Source: CAD feature listing. Evaluate the final solid. Frame: model axes, mm. A direction names the side the tool comes from. Give positions to 0.01 mm unless a question says otherwise; leave off trailing zeros. Loops run counter-clockwise (first coordinate to the right, second up) from the corner with the lowest first, then second, coordinate; pieces in that order, holes last. Notation, with made-up numbers: M 58.25,26 L 77.25,26 A18 ccw 77.25,37 Z; hole C -24,56 d10. An arc over 180 degrees is marked long. Answer in a Markdown table with one row per item.
```python
from build123d import *

# Parameters (mm, degrees)
BOSS_EXTRUDE1_DEPTH = 23.4
SKETCH2_W           = 10.92
SKETCH2_H           = 9.32
BOSS_EXTRUDE2_DEPTH = 1.2
SKETCH3_R           = 1.61
CUT_EXTRUDE1_DEPTH  = 24.4
SKETCH4_R           = 11.05
BOSS_EXTRUDE3_DEPTH = 1.6
SKETCH5_R           = 2.5
BOSS_EXTRUDE4_DEPTH = 11


with BuildPart() as part:
    # Sketch1 → Boss-Extrude1 (new body)
    with BuildSketch(Plane(origin=(0, 0, 0), x_dir=(1, 0, 0), z_dir=(0, 1, 0))):
        Polygon((-17.385, 21.085), (17.385, 21.085), (21.085, 17.385), (21.085, -17.385), (17.385, -21.085), (-17.385, -21.085), (-21.085, -17.385), (-21.085, 17.385), align=None)
    extrude(amount=BOSS_EXTRUDE1_DEPTH)

    # Sketch2 → Boss-Extrude2 (add)
    with BuildSketch(Plane.XY.offset(21.085)):
        with Locations((0, 4.66)):
            Rectangle(SKETCH2_W, SKETCH2_H)
    extrude(amount=BOSS_EXTRUDE2_DEPTH)

    # Sketch3 → Cut-Extrude1 (cut, through all)
    with BuildSketch(Plane(origin=(0, 23.4, 0), x_dir=(1, 0, 0), z_dir=(0, 1, 0))):
        with Locations((-15.37, -15.37)):
            Circle(SKETCH3_R)
        with Locations((15.37, 15.37)):
            Circle(SKETCH3_R)
    extrude(amount=-CUT_EXTRUDE1_DEPTH, mode=Mode.SUBTRACT)

    # Sketch4 → Boss-Extrude3 (add)
    with BuildSketch(Plane(origin=(0, 23.4, 0), x_dir=(1, 0, 0), z_dir=(0, 1, 0))):
        Circle(SKETCH4_R)
    extrude(amount=BOSS_EXTRUDE3_DEPTH)

    # Sketch5 → Boss-Extrude4 (add)
    with BuildSketch(Plane(origin=(0, 25, 0), x_dir=(1, 0, 0), z_dir=(0, 1, 0))):
        Circle(SKETCH5_R)
    extrude(amount=BOSS_EXTRUDE4_DEPTH)


solid = part.part
```
1) Set-up query: faces 5 (the flat face through (-5.46, 5, 22)), 6 (the cylindrical face through (-0.54, 30.42, 2.44)), 7 (the flat face through (5.46, 5, 22)), 8 (the flat face through (0, 9.32, 22)). Return all of +Z, -Z, +X, -X, +Y, -Y with unobstructed straight access to the full face (end or side cutting, diameter ignored); none if empty.
Reply:
| item | result |
|---|---|
| face 5 | +Z, -X, +Y, -Y |
| face 6 | +Y |
| face 7 | +Z, +X, +Y, -Y |
| face 8 | +Z, +X, -X, +Y |
2) Material intervals for L1, parallel to X at y = 5.5, z = -15.37 (3 decimals); L2, parallel to X at y = 5.5, z = 15.37 (3 decimals), sorted ascending.
Reply:
| item | result |
|---|---|
| L1 | x = -21.085 to 13.76, 16.98 to 21.085 |
| L2 | x = -21.085 to -16.98, -13.76 to 21.085 |
3) Section A-A, the plane x = 15.37. Return loops of the section in (y, z) (3 decimals).
Reply:
| item | result |
|---|---|
| outline | M 0,-21.085 L 23.4,-21.085 L 23.4,-16.98 L 0,-16.98 Z; M 0,-13.76 L 23.4,-13.76 L 23.4,21.085 L 0,21.085 Z |
4) Section B-B, the plane y = 2. Return loops of the section in (x, z) (3 decimals).
Reply:
| item | result |
|---|---|
| outline | M -21.085,-17.385 L -17.385,-21.085 L 17.385,-21.085 L 21.085,-17.385 L 21.085,17.385 L 17.385,21.085 L 5.46,21.085 L 5.46,22.285 L -5.46,22.285 L -5.46,21.085 L -17.385,21.085 L -21.085,17.385 Z; hole C -15.37,15.37 d3.22; hole C 15.37,-15.37 d3.22 |
5) Section C-C, the plane z = 15.37. Return loops of the section in (x, y) (3 decimals), then the cut area to 3 significant figures.
Reply:
| item | result |
|---|---|
| outline | M -21.085,0 L -16.98,0 L -16.98,23.4 L -21.085,23.4 Z; M -13.76,0 L 21.085,0 L 21.085,23.4 L -13.76,23.4 Z |
| area | 911 mm² |
6) Pin query (flat end, axial travel): pin 1 Ø1.3 at (y, z) = (6.5, 22) entering from +X; pin 2 Ø5 at (x, z) = (15.37, -15.37) entering from +Y; pin 3 Ø8 at (x, z) = (6.5, -8) entering from +Y; pin 4 Ø24.5 at (x, z) = (2, -2.5) entering from +Y. Return the tip coordinate at first contact, or that it passes through.
Reply:
| item | result |
|---|---|
| pin 1 | stops at x = 5.46 |
| pin 2 | stops at y = 23.4 |
| pin 3 | stops at y = 25 |
| pin 4 | stops at y = 36 |
7) Section D-D, the plane x = 0. Return loops of the section in (y, z) (3 decimals).
Reply:
| item | result |
|---|---|
| outline | M 0,-21.085 L 23.4,-21.085 L 23.4,-11.05 L 25,-11.05 L 25,-2.5 L 36,-2.5 L 36,2.5 L 25,2.5 L 25,11.05 L 23.4,11.05 L 23.4,21.085 L 9.32,21.085 L 9.32,22.285 L 0,22.285 Z |
8) Pull-direction query (Z, two-part tool) for faces 1 (the cylindrical face through (16.236, 11.864, -16.728)), 2 (the flat face through (-9, 23.4, 9)), 3 (the cylindrical face through (-15.58, 11.864, 13.774)), 4 (the flat face through (0, 5, 22.285)); classes: released by +Z, released by -Z, zero draft, split by the parting line, or undercut.
Reply:
| item | result |
|---|---|
| face 1 | undercut |
| face 2 | zero draft |
| face 3 | undercut |
| face 4 | released by +Z |
